from build123d import *

# Parameters (mm, degrees)
F0_W      = 203.2
F0_H      = 101.6
F1_DEPTH  = 12.7
F2_D      = 14.224
F4_W      = 203.2
F4_H      = 101.6
F5_DEPTH  = 12.7
F6_W      = 12.7
F6_H      = 31.75
F6_H_2    = 12.7
F6_W_2    = 31.75
F7_DEPTH  = 263.525
F9_DEPTH  = 25.4
F11_DEPTH = 12.7


with BuildPart() as f1:
    # F0 (on Top) → F1 (new body)
    with BuildSketch(Plane.XY):
        Rectangle(F0_W, F0_H)
    extrude(amount=-F1_DEPTH)

    # F2 (through all)
    with Locations(Plane.XY):
        with Locations((-76.2, 25.4), (76.2, 25.4), (76.2, -25.4), (-76.2, -25.4)):
            Hole(F2_D / 2)



with BuildPart() as f5:
    # F4 (on offset) → F5 (new body)
    with BuildSketch(Plane(origin=(0, 0, 276.225), x_dir=(1, 0, 0), z_dir=(0, 0, -1))):
        Rectangle(F4_W, F4_H)
    extrude(amount=F5_DEPTH)

    # F8 (on face) → F9 (cut)
    with BuildSketch(Plane.XY.offset(276.225)):
        with BuildLine():
            Line((-54.76875, -12.7), (-54.76875, 12.7))
            ThreePointArc((-54.76875, 12.7), (-60.325, 7.14375), (-65.88125, 12.7))
            Line((-65.88125, 12.7), (-65.88125, -12.7))
            ThreePointArc((-65.88125, -12.7), (-60.325, -7.14375), (-54.76875, -12.7))
        make_face()
        with BuildLine():
            ThreePointArc((-65.88125, 12.7), (-60.325, 7.14375), (-54.76875, 12.7))
            Line((-54.76875, 12.7), (-54.76875, 38.1))
            ThreePointArc((-54.76875, 38.1), (-60.325, 43.65625), (-65.88125, 38.1))
            Line((-65.88125, 38.1), (-65.88125, 12.7))
        make_face()
        with BuildLine():
            Line((-54.76875, -38.1), (-54.76875, -12.7))
            ThreePointArc((-54.76875, -12.7), (-60.325, -7.14375), (-65.88125, -12.7))
            Line((-65.88125, -12.7), (-65.88125, -38.1))
            ThreePointArc((-65.88125, -38.1), (-60.325, -43.65625), (-54.76875, -38.1))
        make_face()
        with BuildLine():
            Line((54.76875, 12.7), (54.76875, -12.7))
            ThreePointArc((54.76875, -12.7), (60.325, -7.14375), (65.88125, -12.7))
            Line((65.88125, -12.7), (65.88125, 12.7))
            ThreePointArc((65.88125, 12.7), (60.325, 7.14375), (54.76875, 12.7))
        make_face()
        with BuildLine():
            ThreePointArc((65.88125, -12.7), (60.325, -7.14375), (54.76875, -12.7))
            Line((54.76875, -12.7), (54.76875, -38.1))
            ThreePointArc((54.76875, -38.1), (60.325, -43.65625), (65.88125, -38.1))
            Line((65.88125, -38.1), (65.88125, -12.7))
        make_face()
        with BuildLine():
            Line((54.76875, 38.1), (54.76875, 12.7))
            ThreePointArc((54.76875, 12.7), (60.325, 7.14375), (65.88125, 12.7))
            Line((65.88125, 12.7), (65.88125, 38.1))
            ThreePointArc((65.88125, 38.1), (60.325, 43.65625), (54.76875, 38.1))
        make_face()
    extrude(amount=-F9_DEPTH, mode=Mode.SUBTRACT)


with BuildPart() as f7:
    # F6 (on face) → F7 (new body, through all)
    with BuildSketch(Plane.XY):
        with Locations((0, 22.225)):
            Rectangle(F6_W, F6_H)
        Rectangle(F6_W, F6_H_2)
        with Locations((-22.225, 0)):
            Rectangle(F6_W_2, F6_H_2)
        with Locations((22.225, 0)):
            Rectangle(F6_W_2, F6_H_2)
        with Locations((0, -22.225)):
            Rectangle(F6_W, F6_H)
    extrude(amount=F7_DEPTH)


with BuildPart() as f1_1:
    add(f1.part)

    add(f5.part)  # F11 merges F5

    add(f7.part)  # F11 merges F7
    # F10 (on face) → F11 (join)
    with BuildSketch(Plane.XZ.offset(6.35)):
        Polygon((88.9, 0), (38.1, 263.5250000004), (38.1, 7e-10), align=None)
        Polygon((-88.9, 0), (-38.1, 0), (-38.1, 263.5250000004), align=None)
    extrude(amount=-F11_DEPTH)


solid = f1_1.part
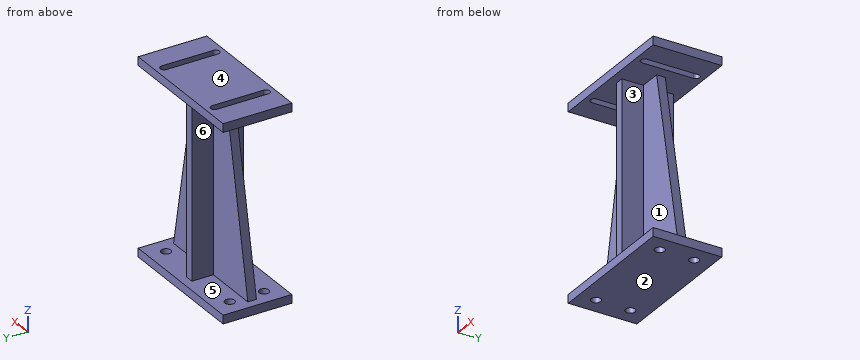
For this review, take the finished solid that the model builds, in its own axes (mm). Face numbers are marked on the shaded views. A direction names the side the tool comes from. Round coordinates to 2 decimals unless told otherwise and drop trailing zeros. Write each loop counter-clockwise with the first axis right and the second up, starting at its lowest first coordinate (ties: lowest second). Pieces come first, ordered by that corner, then holes. Notation, with made-up numbers: (-31.5, -12.75) -> (-17.5, -12.75) arc R10 ccw to (-17.5, 5.25) -> close; hole circle Ø9 at (2, 23.5). An arc over 180 degrees is marked (long way). Put each result on its own line as item: value.
Q1. The part is to be moulded in two halves that separate along Z. For the marked faces 1, 2, 3 and 4, say which applies: released by +Z, released by -Z, zero draft, split by the parting line, or undercut.
Determined:
face 1: undercut
face 2: released by -Z
face 3: undercut
face 4: released by +Z
Q2. Consider section C-C on y = -25.4. State the section outline as (x, z) points (3 decimals).
Determined:
outline: (-101.6, -12.7) -> (-83.312, -12.7) -> (-83.312, 0) -> (-101.6, 0) -> close; (-101.6, 263.525) -> (-65.881, 263.525) -> (-65.881, 276.225) -> (-101.6, 276.225) -> close; (-69.088, -12.7) -> (69.088, -12.7) -> (69.088, 0) -> (6.35, 0) -> (6.35, 263.525) -> (54.769, 263.525) -> (54.769, 276.225) -> (-54.769, 276.225) -> (-54.769, 263.525) -> (-6.35, 263.525) -> (-6.35, 0) -> (-69.088, 0) -> close; (65.881, 263.525) -> (101.6, 263.525) -> (101.6, 276.225) -> (65.881, 276.225) -> close; (83.312, -12.7) -> (101.6, -12.7) -> (101.6, 0) -> (83.312, 0) -> close
Q3. Consider section D-D on x = 29. State the section outline as (y, z) points (3 decimals), and give its area (3 significant figures).
Determined:
outline: (-50.8, -12.7) -> (50.8, -12.7) -> (50.8, 0) -> (6.35, 0) -> (6.35, 263.525) -> (50.8, 263.525) -> (50.8, 276.225) -> (-50.8, 276.225) -> (-50.8, 263.525) -> (-6.35, 263.525) -> (-6.35, 0) -> (-50.8, 0) -> close
area: 5,930 mm^2
Q4. Clearance check with flat-ended pins moving along their axes: pin 1 Ø9.5 at (y, z) = (28, 101) entering from +X; pin 2 Ø12 at (y, z) = (35, 161.5) entering from -X; pin 3 Ø2 at (x, z) = (-11, 115.5) entering from +Y. State where each tip first meets the part, or that it passes through.
Determined:
pin 1: stops at x = 6.35
pin 2: stops at x = -6.35
pin 3: stops at y = 6.35
Q5. Consider section A-A on x = 76.2. State the section outline as (y, z) points (3 decimals), and give its area (3 significant figures).
Determined:
outline: (-50.8, -12.7) -> (-32.512, -12.7) -> (-32.512, 0) -> (-50.8, 0) -> close; (-50.8, 263.525) -> (50.8, 263.525) -> (50.8, 276.225) -> (-50.8, 276.225) -> close; (-18.288, -12.7) -> (18.288, -12.7) -> (18.288, 0) -> (6.35, 0) -> (6.35, 65.881) -> (-6.35, 65.881) -> (-6.35, 0) -> (-18.288, 0) -> close; (32.512, -12.7) -> (50.8, -12.7) -> (50.8, 0) -> (32.512, 0) -> close
area: 3,060 mm^2
Q6. Machinability: for the marked faces 5 and 6, which of the approach directions +Z, -Z, +X, -X, +Y, -Y give a long, thin tool a straight path to every point of the face, cutting with its end or side? Answer none if there is none.
Determined:
face 5: none
face 6: -X, +Y
Q7. To check wall thickness, follow L1, parallel to Y at x = -76.2, z = -6.5; L2, parallel to X at y = 25, z = -9; L3, parallel to Z at x = -86, y = 10.5 (3 decimals). State the ranges of each line that lie inside material, in increasing order. Write a range as [from, to].
Determined:
L1: y = [-50.8, -32.51], [-18.29, 18.29], [32.51, 50.8]
L2: x = [-101.6, -83.3], [-69.1, 69.1], [83.3, 101.6]
L3: z = [-12.7, 0], [263.525, 276.225]
Q8. Consider section B-B on y = 1. State the section outline as (x, z) points (3 decimals).
Determined:
outline: (-101.6, -12.7) -> (101.6, -12.7) -> (101.6, 0) -> (88.9, 0) -> (38.1, 263.525) -> (54.769, 263.525) -> (54.769, 276.225) -> (-54.769, 276.225) -> (-54.769, 263.525) -> (-38.1, 263.525) -> (-88.9, 0) -> (-101.6, 0) -> close; (-101.6, 263.525) -> (-65.881, 263.525) -> (-65.881, 276.225) -> (-101.6, 276.225) -> close; (65.881, 263.525) -> (101.6, 263.525) -> (101.6, 276.225) -> (65.881, 276.225) -> close
